Geometry: final body of the model. Coordinates: model frame, mm. Face numbers are marked on the shaded views. A direction names the side the tool comes from. Give positions to 0.01 mm unless a question says otherwise; leave off trailing zeros. Loops run counter-clockwise (first coordinate to the right, second up) from the corner with the lowest first, then second, coordinate; pieces in that order, holes last.
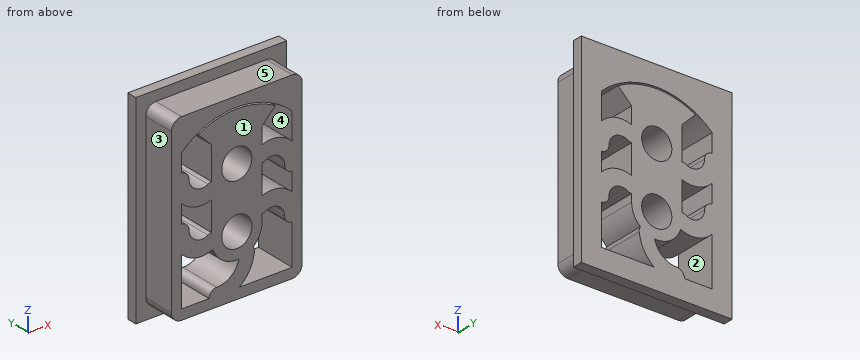
from build123d import *

# Parameters (mm, degrees)
SKETCH1_W           = 13
SKETCH1_H           = 18
BOSS_EXTRUDE1_DEPTH = 3.2
SKETCH2_W           = 15
SKETCH2_H           = 20
BOSS_EXTRUDE2_DEPTH = 1
SKETCH4_R           = 1.5
CUT_EXTRUDE2_DEPTH  = 14.18673576
FILLET1_R           = 1


with BuildPart() as part:
    # Sketch1 → Boss-Extrude1 (new body)
    with BuildSketch(Plane(origin=(0, 0, 0), x_dir=(1, 0, 0), z_dir=(0, 1, 0))):
        Rectangle(SKETCH1_W, SKETCH1_H)
    extrude(amount=BOSS_EXTRUDE1_DEPTH)

    # Sketch2 → Boss-Extrude2 (add)
    with BuildSketch(Plane(origin=(0, 3.2, 0), x_dir=(1, 0, 0), z_dir=(0, 1, 0))):
        Rectangle(SKETCH2_W, SKETCH2_H)
    extrude(amount=BOSS_EXTRUDE2_DEPTH)

    # Sketch4 → Cut-Extrude2 (cut, through all)
    with BuildSketch(Plane.XZ):
        with BuildLine():
            Line((-2.5, 5.5), (-3.844272635, 6.844272635))
            ThreePointArc((-3.844272635, 6.844272635), (0, 7.85), (3.844272635, 6.844272635))
            Line((3.844272635, 6.844272635), (2.5, 5.5))
            Line((2.5, 5.5), (2.5, 2.25))
            ThreePointArc((2.5, 2.25), (2.694114284, 2.22444437), (2.875, 2.149519053))
            ThreePointArc((2.875, 2.149519053), (4.125, 2.149519053), (4.75, 3.232050808))
            ThreePointArc((4.75, 3.232050808), (4.969669914, 3.762380893), (5.5, 3.982050808))
            Line((5.5, 3.982050808), (5.5, 5.809475019))
            ThreePointArc((5.5, 5.809475019), (0, 8), (-5.5, 5.809475019))
            Line((-5.5, 5.809475019), (-5.5, 3.155407801))
            ThreePointArc((-5.5, 3.155407801), (-4.103044833, 3.951014031), (-2.5, 3.829686884))
            Line((-2.5, 3.829686884), (-2.5, 5.5))
        make_face()
        with Locations(Location((0, 3, 0), (0, 0, 270))):
            Circle(SKETCH4_R)
        with BuildLine():
            Line((-2.5, -0.670313116), (-2.5, 2.25))
            ThreePointArc((-2.5, 2.25), (-2.694114284, 2.27555563), (-2.875, 2.350480947))
            ThreePointArc((-2.875, 2.350480947), (-4.125, 2.350480947), (-4.75, 1.267949192))
            ThreePointArc((-4.75, 1.267949192), (-4.969669914, 0.737619107), (-5.5, 0.517949192))
            Line((-5.5, 0.517949192), (-5.5, -1.344592199))
            ThreePointArc((-5.5, -1.344592199), (-4.103044833, -0.548985969), (-2.5, -0.670313116))
        make_face()
        with BuildLine():
            ThreePointArc((5.5, 1.344592199), (4.103044833, 0.548985969), (2.5, 0.670313116))
            Line((2.5, 0.670313116), (2.5, -2.25))
            ThreePointArc((2.5, -2.25), (2.694114284, -2.27555563), (2.875, -2.350480947))
            ThreePointArc((2.875, -2.350480947), (4.125, -2.350480947), (4.75, -1.267949192))
            ThreePointArc((4.75, -1.267949192), (4.969669914, -0.737619107), (5.5, -0.517949192))
            Line((5.5, -0.517949192), (5.5, 1.344592199))
        make_face()
        with Locations(Location((0, -3, 0), (0, 0, 270))):
            Circle(SKETCH4_R)
        with BuildLine():
            Line((-2.5, -3), (-2.5, -2.25))
            ThreePointArc((-2.5, -2.25), (-2.694114284, -2.22444437), (-2.875, -2.149519053))
            ThreePointArc((-2.875, -2.149519053), (-4.125, -2.149519053), (-4.75, -3.232050808))
            ThreePointArc((-4.75, -3.232050808), (-4.969669914, -3.762380893), (-5.5, -3.982050808))
            Line((-5.5, -3.982050808), (-5.5, -8))
            Line((-5.5, -8), (-0.25521468, -8))
            ThreePointArc((-0.25521468, -8), (-1.276630283, -6.840114098), (-1.746104794, -5.367626807))
            ThreePointArc((-1.746104794, -5.367626807), (-1.730239257, -5.120259699), (-1.634609263, -4.891574095))
            ThreePointArc((-1.634609263, -4.891574095), (-2.27338109, -4.040066547), (-2.5, -3))
        make_face()
        with BuildLine():
            ThreePointArc((5.5, -3.155407801), (4.037255458, -3.964958012), (2.375948891, -3.777731873))
            ThreePointArc((2.375948891, -3.777731873), (1.381615815, -5.083539714), (-0.208211888, -5.491314474))
            ThreePointArc((-0.208211888, -5.491314474), (0.58851368, -6.756605145), (2, -7.25))
            ThreePointArc((2, -7.25), (2.530330086, -7.469669914), (2.75, -8))
            Line((2.75, -8), (5.5, -8))
            Line((5.5, -8), (5.5, -3.155407801))
        make_face()
    extrude(amount=-CUT_EXTRUDE2_DEPTH, mode=Mode.SUBTRACT)

    # Fillet1
    fillet1_edges = [part.edges().sort_by_distance(p)[0] for p in [
        (6.5, 1.6, 9),
        (-6.5, 1.6, 9),
        (-6.5, 1.6, -9),
        (6.5, 1.6, -9),
    ]]
    fillet(fillet1_edges, radius=FILLET1_R)


with BuildPart() as body_2:
    # Mirror2: mirrored copy
    add(part.part.mirror(Plane(origin=(7.5, 4.2, 10), x_dir=(0, 0, 1), z_dir=(-1, 0, 0))))


solid = body_2.part
Item 1: Ray query, probe 1 along X at (y, z) = (3.05, 0.25); probe 2 along Z at (x, y) = (10.75, 2.7); probe 3 along X at (y, z) = (2.1, -5). Return the intervals inside material, ascending.
Values follow:
probe 1: x = 8.5 to 9.5, 12.5 to 17.5, 20.5 to 21.5
probe 2: z = -9 to -8, -3.91 to -2.27, 0.59 to 2.23, 6.78 to 9
probe 3: x = 8.5 to 9.5, 13.5 to 16.69, 20.5 to 21.5
Item 2: Section query B-B on z = -3.5. Return loops of the section in (x, y), plus the area to 3 significant figures.
Values follow:
outline: (7.5, 3.2) - (8.5, 3.2) - (8.5, 0) - (9.5, 0) - (9.5, 4.2) - (7.5, 4.2) - close; (9.89, 0) - (13.59, 0) - (13.59, 4.2) - (9.89, 4.2) - close; (16.41, 0) - (17.45, 0) - (17.45, 4.2) - (16.41, 4.2) - close; (19.8, 0) - (21.5, 0) - (21.5, 3.2) - (22.5, 3.2) - (22.5, 4.2) - (19.8, 4.2) - close
area: 33.2 mm2
Item 3: Draft query along Z for the marked faces 3, 4 and 5. Return one class per face: +Z half, -Z half, draft (parallel to the pull), parting line (faces both ways), or undercut.
Values follow:
face 3: draft
face 4: undercut
face 5: +Z half
Item 4: Section query A-A on x = 19.25. Return loops of the section in (y, z), plus the area to 3 significant figures.
Values follow:
outline: (0, -9) - (3.2, -9) - (3.2, -10) - (4.2, -10) - (4.2, -8) - (0, -8) - close; (0, -2.23) - (4.2, -2.23) - (4.2, -0.59) - (0, -0.59) - close; (0, 2.27) - (4.2, 2.27) - (4.2, 3.91) - (0, 3.91) - close; (0, 6.78) - (4.2, 6.78) - (4.2, 10) - (3.2, 10) - (3.2, 9) - (0, 9) - close
area: 29.4 mm2
Item 5: Set-up query: the marked faces 1 and 2. Return all of +Z, -Z, +X, -X, +Y, -Y with unobstructed straight access to the full face (end or side cutting, diameter ignored); none if empty.
Values follow:
face 1: +Z, -Z, +X, -X, -Y
face 2: +Y, -Y
Item 6: Section query C-C on x = 14. Return loops of the section in (y, z), plus the area to 3 significant figures.
Values follow:
outline: (0, -9) - (3.2, -9) - (3.2, -10) - (4.2, -10) - (4.2, -7.02) - (0, -7.02) - close; (0, -5.29) - (4.2, -5.29) - (4.2, -4.12) - (0, -4.12) - close; (0, -1.88) - (4.2, -1.88) - (4.2, 1.88) - (0, 1.88) - close; (0, 4.12) - (4.2, 4.12) - (4.2, 7.79) - (0, 7.79) - close; (0, 7.94) - (4.2, 7.94) - (4.2, 10) - (3.2, 10) - (3.2, 9) - (0, 9) - close
area: 50.9 mm2
Item 7: Section query D-D on y = 3.55. Give the number of separate pieces and of enclosed holes in the cut face, plus the area to 3 significant figures.
Values follow:
separate pieces: 1
enclosed holes: 7
area: 212 mm2
Item 8: Pin query (flat end, axial travel): pin 1 (1.6 mm diameter, centred on y = 1.5, z = 3.5, fed in from -X); pin 2 (1 mm diameter, centred on x = 20, z = -2.5, fed in from -Y); pin 3 (2 mm diameter, centred on y = 1, z = 7, fed in from +X); pin 4 (1.3 mm diameter, centred on x = 17.5, y = 2, fed in from +Z). Return the tip coordinate at first contact, or that it passes through.
Values follow:
pin 1: stops at x = 8.5
pin 2: stops at y = 0
pin 3: stops at x = 21.5
pin 4: stops at z = 9
